For this review, take the finished solid that the model builds, in its own axes (mm). A direction names the side the tool comes from. Round coordinates to 2 decimals unless told otherwise and drop trailing zeros. Write each loop counter-clockwise with the first axis right and the second up, starting at its lowest first coordinate (ties: lowest second). Pieces come first, ordered by that corner, then holes. Notation, with made-up numbers: M 29.5,63 L 35.5,63 A22 cw 35.5,82 Z; hole C 14.5,-16 d6. An arc over 180 degrees is marked long. Use one line per item in the form item = value. Start each with the question number.
Item 1: Draft analysis for pull direction Y (two halves, no side actions). For faces 1 (the flat face through (-3, -16, 9)), 2 (the flat face through (-3, 0, 1)), 3 (the flat face through (-3, -400, 1)), state which applies: released by +Y, released by -Y, zero draft, split by the parting line, or undercut.
Item 2: For line 1 (X direction, y = -196, z = 2.5); line 2 (Y direction, x = 38.5, z = -54.5); line 3 (Y direction, x = 124, z = -89.25), list the stretches that pass through material, from the lowest coordinate up. Write a range as [from, to].
Item 3: For faces 4 (the flat face through (-200, -197, -1)), 5 (the cylindrical face through (1.953, -8.112, 25.128)), 6 (the flat face through (-3, -384, 9)), list the 3-axis set-ups (+Z, -Z, +X, -X, +Y, -Y) from which the entire face can be reached by the end or side of a thin tool; tool diameter is ignored.
Item 4: Add section C-C (z = -60). State the section outline as (x, y) points, and give its area (3 significant figures).
Item 5: For P1, Ø4, axis at x = -93.5, y = -134, coming from the +Z side, flat-tipped, find the tip position at first contact; note if it passes through.
Item 6: Add section D-D (x = 50.5). State the section outline as (y, z) points, and give its area (3 significant figures).
Item 7: Add section A-A (x = 0). State the section outline as (y, z) points.
Item 8: Add section B-B (y = -324). State the section outline as (x, z) points.
from build123d import *

# Parameters (mm, degrees)
F0_W     = 400
F0_H     = 200
F1_DEPTH = 400
F2_T     = -16
F3_D     = 30
F3_DEPTH = 16
F3_TIP   = 9.0129092854
F5_D     = 50


with BuildPart() as f1:
    # F0 (on Front) → F1 (new body)
    with BuildSketch(Plane.XZ):
        Rectangle(F0_W, F0_H)
    extrude(amount=F1_DEPTH)

    # F2
    f2_openings = [f1.faces().sort_by_distance(p)[0] for p in [
        (0, -200, 100),
    ]]
    offset(amount=F2_T, openings=f2_openings)

    # F3
    with Locations(Plane(origin=(0, 0, 0), x_dir=(1, 0, 0), z_dir=(0, 1, 0))):
        with Locations((0, -40)):
            Hole(F3_D / 2, depth=F3_DEPTH)
            with Locations((0, 0, -(F3_DEPTH + F3_TIP / 2))):  # 118° drill point
                Cone(0, F3_D / 2, F3_TIP, mode=Mode.SUBTRACT)

    # F5 (through all)
    with Locations(Plane.XY.offset(-84)):
        with Locations((124, -324)):
            Hole(F5_D / 2)


solid = f1.part
Calculated:
q1.face_1 = undercut
q1.face_2 = released by +Y
q1.face_3 = released by -Y
q2.line_1 = [-200, -184], [184, 200]
q2.line_2 = [-400, -384], [-16, 0]
q2.line_3 = [-400, -349], [-299, 0]
q3.face_4 = +Z, -Z, -X, +Y, -Y
q3.face_5 = +Y
q3.face_6 = +Z
q4.outline = M -200,-400 L 200,-400 L 200,0 L -200,0 Z; hole M -184,-384 L 184,-384 L 184,-16 L -184,-16 Z
q4.area = 24,600 mm^2
q5.P1 = -84
q6.outline = M -400,-100 L 0,-100 L 0,100 L -16,100 L -16,-84 L -384,-84 L -384,100 L -400,100 Z
q6.area = 12,300 mm^2
q7.outline = M -400,-100 L 0,-100 L 0,25 L -16,25 L -16,-84 L -384,-84 L -384,100 L -400,100 Z; M -16,55 L 0,55 L 0,100 L -16,100 Z
q8.outline = M -200,-100 L 99,-100 L 99,-84 L -184,-84 L -184,100 L -200,100 Z; M 149,-100 L 200,-100 L 200,100 L 184,100 L 184,-84 L 149,-84 Z
